Could you check a few things on this drawing? It's one solid part, dimensions in mm from its lowest x, y, z. A direction names the side the tool comes from. Round coordinates to 2 decimals unless told otherwise and drop trailing zeros. Loops run counter-clockwise (first coordinate to the right, second up) from the corner with the lowest first, then second, coordinate; pieces in that order, holes last. Notation, with made-up numbers: M 39.5,55 L 70.5,55 A26 ccw 70.5,84 Z; hole C 62.5,89.25 d2. An arc over 180 degrees is marked long. Put each result on its own line as item: value. Start each with the question number.
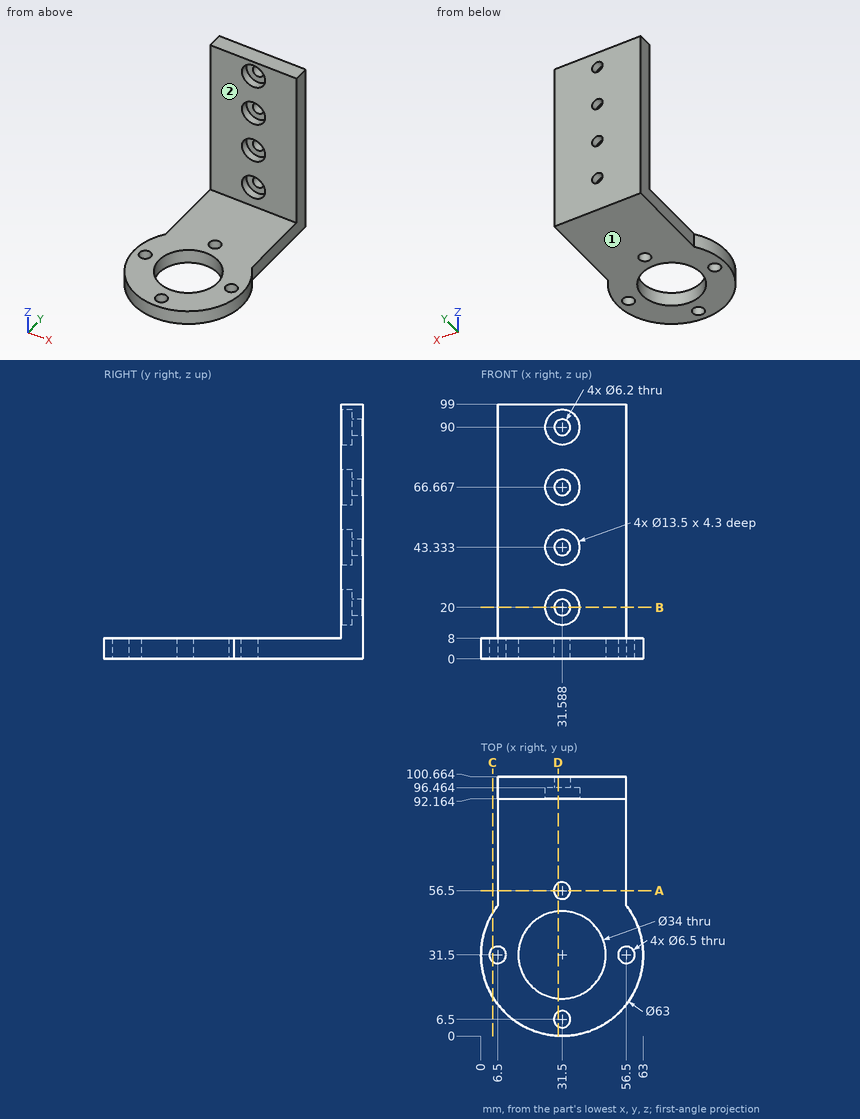
1) On a 3-axis mill with a long thin cutter (end or side, diameter ignored), from which of +Z, -Z, +X, -X, +Y, -Y can I reach the whole of each face in a straight line? I mean the marked faces 1 and 2. Say none if no direction works.
2) Suppose I cut it at C-C (x = 4.5). Write out the boundary of the cut face in (y, z) (1 decimal).
3) Suppose I cut it at B-B (z = 20). Write out the boundary of the cut face in (x, y).
4) Suppose I cut it at D-D (x = 30). State how many separate pieces and enclosed holes the cut face has.
5) I'm going to push flat-ended pins straight in: P1, Ø15, axis at x = 34.5, z = 91.5, coming from the -Y side; P2, Ø3.5, axis at x = 31.59, z = 66.67, coming from the +Y side; P3, Ø10, axis at x = 16, y = 47, coming from the +Z side. Where does each tip first touch, or does it pass through?
6) If I drill on probe 1 along X at (y, z) = (97.5, 20); probe 2 along Z at (x, y) = (15.5, 45.5); probe 3 along Y at (x, z) = (32, 84), over which ranges is the centre line in solid material (lowest first)? Write a range as from..to.
7) Suppose I cut it at A-A (y = 56.5). Write out the boundary of the cut face in (x, z), plus the area to 3 significant figures.
Results are:
1. face 1: -Z, +X, -X, +Y, -Y
1. face 2: +Z, +X, -X, -Y
2. outline: M 15.3,0 L 28.9,0 L 28.9,8 L 15.3,8 Z; M 34.1,0 L 47.7,0 L 47.7,8 L 34.1,8 Z
3. outline: M 6.5,92.16 L 24.84,92.16 L 24.84,96.46 L 28.49,96.46 L 28.49,100.66 L 6.5,100.66 Z; M 34.69,96.46 L 38.34,96.46 L 38.34,92.16 L 56.5,92.16 L 56.5,100.66 L 34.69,100.66 Z
4. separate pieces: 8
4. enclosed holes: 0
5. P1: y = 92.16
5. P2: through
5. P3: z = 8
6. probe 1: 6.5..28.49, 34.69..56.5
6. probe 2: 0..8
6. probe 3: 96.46..100.66
7. outline: M 6.5,0 L 28.25,0 L 28.25,8 L 6.5,8 Z; M 34.75,0 L 56.5,0 L 56.5,8 L 34.75,8 Z
7. area: 348 mm²
